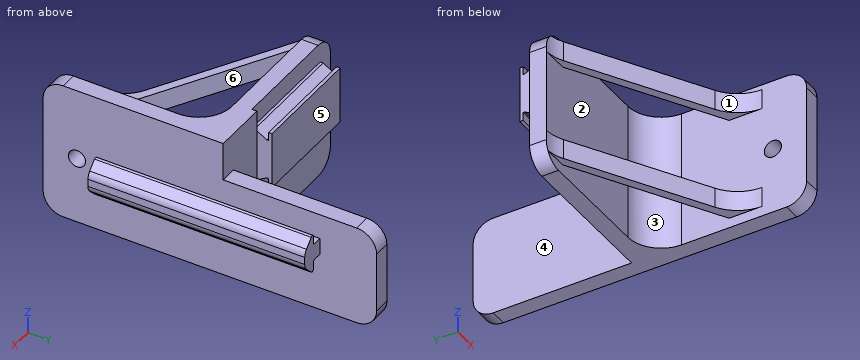
```python
from build123d import *

# Parameters (mm, degrees)
BOSS_EXTRUDE5_DEPTH  = 50
SKETCH11_W           = 41.5
SKETCH11_H           = 100
BOSS_EXTRUDE6_DEPTH  = 5
SKETCH12_W           = 41.5
SKETCH12_H           = 5
BOSS_EXTRUDE8_DEPTH  = 55
SKETCH13_W           = 11.5
SKETCH13_H           = 47.5
CUT_EXTRUDE1_DEPTH   = 55
BOSS_EXTRUDE9_DEPTH  = 6
FILLET7_R            = 12
FILLET7_OF_MIRROR1_R = 12
FILLET8_R            = 6
BOSS_EXTRUDE10_START = 8
BOSS_EXTRUDE10_DEPTH = 8
FILLET12_R           = 10
BOSS_EXTRUDE11_DEPTH = 57
SKETCH16_R           = 2.575
CUT_EXTRUDE2_DEPTH   = 10
SKETCH17_W           = 27.480150942
SKETCH17_H           = 1.5
BOSS_EXTRUDE12_DEPTH = 11.5
SKETCH18_W           = 11.5
SKETCH18_H           = 1.5
BOSS_EXTRUDE13_DEPTH = 5
BOSS_EXTRUDE14_START = -5
BOSS_EXTRUDE14_DEPTH = 33.5


with BuildPart() as part:
    # Sketch9 → Boss-Extrude5 (new body)
    with BuildSketch(Plane(origin=(0, 245, 0), x_dir=(1, 0, 0), z_dir=(0, 1, 0))):
        with BuildLine():
            Line((389.629800237, -111.599739584), (387.629800237, -111.599739584))
            Line((387.629800237, -111.599739584), (387.629800237, -106.649739584))
            Line((387.629800237, -106.649739584), (389.629800237, -106.649739584))
            Line((389.629800237, -106.649739584), (390.329799474, -106.649739584))
            ThreePointArc((390.329799474, -106.649739584), (390.605571069, -106.535511279), (390.719799474, -106.259739725))
            Line((390.719799474, -106.259739725), (390.719800256, -104.090618139))
            ThreePointArc((390.719800256, -104.090618139), (391.145748802, -103.453141463), (391.897703935, -103.602714709))
            Line((391.897703935, -103.602714709), (394.237480965, -105.942491739))
            ThreePointArc((394.237480965, -105.942491739), (394.868289671, -106.886563682), (395.089800232, -108.000172467))
            Line((395.089800232, -108.000172467), (395.089800237, -110.249306685))
            ThreePointArc((395.089800237, -110.249306685), (394.868289678, -111.362915477), (394.23748097, -112.306987424))
            Line((394.23748097, -112.306987424), (391.897703941, -114.646764454))
            ThreePointArc((391.897703941, -114.646764454), (391.145748809, -114.7963377), (390.719800262, -114.158861025))
            Line((390.719800262, -114.158861025), (390.719799474, -111.989739443))
            ThreePointArc((390.719799474, -111.989739443), (390.605571069, -111.71396789), (390.329799474, -111.599739584))
            Line((390.329799474, -111.599739584), (389.629800237, -111.599739584))
        make_face()
    extrude(amount=-BOSS_EXTRUDE5_DEPTH)

    # Sketch11 → Boss-Extrude6 (add)
    with BuildSketch(Plane.ZY.offset(-387.629800242)):
        with Locations((109.874739584, 220)):
            Rectangle(SKETCH11_W, SKETCH11_H)
    extrude(amount=BOSS_EXTRUDE6_DEPTH)

    # Sketch12 → Boss-Extrude8 (add)
    with BuildSketch(Plane.ZY.offset(-387.629800242)):
        with Locations((109.874739584, 220)):
            Rectangle(SKETCH12_W, SKETCH12_H)
    extrude(amount=BOSS_EXTRUDE8_DEPTH)

    # Sketch13 → Cut-Extrude1 (cut)
    with BuildSketch(Plane.ZY.offset(-387.629800242)):
        with Locations((124.874739584, 246.25)):
            Rectangle(SKETCH13_W, SKETCH13_H)
    extrude(amount=CUT_EXTRUDE1_DEPTH, mode=Mode.SUBTRACT)

    # Sketch15 → Boss-Extrude9 (add)
    with BuildSketch(Plane.XY.offset(129.124739584)):
        Polygon((335.629800242, 217.5), (382.629800242, 190.364537348), (382.629800242, 193.251288694), (340.629800242, 217.5), align=None)
    boss_extrude9 = extrude(amount=-BOSS_EXTRUDE9_DEPTH)

    # Fillet7
    # the kernel refuses this fillet: 12 mm, written as the material it adds along each edge
    with BuildSketch(Plane(origin=(335.629800242, 217.5, 129.124739584), x_dir=(-1, 0, 0), z_dir=(0, 0, -1))) as fillet7_piece_1:
        with BuildLine():
            CenterArc((3.218847051, -11.998004249), FILLET7_R, 91.044975628, 28.955024372)
            Line((-2.781152949, -1.605699404), (-2.901152949, -1.397853307))
            Line((-2.901152949, -1.397853307), (-0.12, 0.207846097))
            Line((-0.12, 0.207846097), (0, 0.24))
            ThreePointArc((0, 0.24), (1.5, 0.24), (2.995623059, 0.239960085))
            Line((2.995623059, 0.239960085), (3, 0))
        make_face()
    extrude(amount=6)
    with BuildSketch(Plane(origin=(382.629800242, 190.364537348, 129.124739584), x_dir=(0, -1, 0), z_dir=(0, 0, -1))) as fillet7_piece_2:
        with BuildLine():
            CenterArc((FILLET7_R * 0.57735026919, FILLET7_R), FILLET7_R, 210, 60)
            Line((-FILLET7_R * 0.288675134595, FILLET7_R * 0.5), (-FILLET7_R * 0.305995642671, FILLET7_R * 0.49))
            Line((-FILLET7_R * 0.305995642671, FILLET7_R * 0.49), (-FILLET7_R * 0.0115470053838, -FILLET7_R * 0.02))
            Line((-FILLET7_R * 0.0115470053838, -FILLET7_R * 0.02), (FILLET7_R * 0.57735026919, -FILLET7_R * 0.02))
            Line((FILLET7_R * 0.57735026919, -FILLET7_R * 0.02), (FILLET7_R * 0.57735026919, 0))
        make_face()
    extrude(amount=6)

    # Mirror1: Boss-Extrude9 across plane
    add(boss_extrude9.mirror(Plane.XY.offset(110.624739584)))

    # Fillet7 of Mirror1
    # the kernel refuses this fillet: 12 mm, written as the material it adds along each edge
    with BuildSketch(Plane(origin=(335.629800242, 217.5, 92.124739584), x_dir=(-1, 0, 0), z_dir=(0, 0, 1))) as fillet7_of_mirror1_piece_1:
        with BuildLine():
            CenterArc((3.218847051, 11.998004249), FILLET7_OF_MIRROR1_R, 240, 28.955024372)
            Line((-2.781152949, 1.605699404), (-2.901152949, 1.397853307))
            Line((-2.901152949, 1.397853307), (-0.12, -0.207846097))
            Line((-0.12, -0.207846097), (0, -0.24))
            ThreePointArc((0, -0.24), (1.5, -0.24), (2.995623059, -0.239960085))
            Line((2.995623059, -0.239960085), (3, 0))
        make_face()
    extrude(amount=6)
    with BuildSketch(Plane(origin=(382.629800242, 190.364537348, 92.124739584), x_dir=(0, -1, 0), z_dir=(0, 0, 1))) as fillet7_of_mirror1_piece_2:
        with BuildLine():
            CenterArc((FILLET7_OF_MIRROR1_R * 0.57735026919, -FILLET7_OF_MIRROR1_R), FILLET7_OF_MIRROR1_R, 90, 60)
            Line((-FILLET7_OF_MIRROR1_R * 0.288675134595, -FILLET7_OF_MIRROR1_R * 0.5), (-FILLET7_OF_MIRROR1_R * 0.305995642671, -FILLET7_OF_MIRROR1_R * 0.49))
            Line((-FILLET7_OF_MIRROR1_R * 0.305995642671, -FILLET7_OF_MIRROR1_R * 0.49), (-FILLET7_OF_MIRROR1_R * 0.0115470053838, FILLET7_OF_MIRROR1_R * 0.02))
            Line((-FILLET7_OF_MIRROR1_R * 0.0115470053838, FILLET7_OF_MIRROR1_R * 0.02), (FILLET7_OF_MIRROR1_R * 0.57735026919, FILLET7_OF_MIRROR1_R * 0.02))
            Line((FILLET7_OF_MIRROR1_R * 0.57735026919, FILLET7_OF_MIRROR1_R * 0.02), (FILLET7_OF_MIRROR1_R * 0.57735026919, 0))
        make_face()
    extrude(amount=6)

    # Fillet8
    # the kernel refuses this fillet: 6 mm, written as the material it takes off along each edge
    with BuildSketch(Plane(origin=(402.629800242, 270, 89.124739584), x_dir=(0, 0, 1), z_dir=(-1, 0, 0)), Plane(origin=(332.629800242, 237.5, 89.124739584), x_dir=(0, 0, 1), z_dir=(0, -1, 0)), Plane(origin=(402.629800242, 270, 119.124739584), x_dir=(0, -1, 0), z_dir=(-1, 0, 0))) as fillet8_piece_1:
        with BuildLine():
            CenterArc((FILLET8_R, -FILLET8_R), FILLET8_R, 90, 90)
            Line((0, -FILLET8_R), (0, 0))
            Line((0, 0), (FILLET8_R, 0))
        make_face()
    extrude(amount=35, mode=Mode.SUBTRACT)
    with BuildSketch(Plane(origin=(402.629800242, 170, 89.124739584), x_dir=(0, 0, 1), z_dir=(-1, 0, 0)), Plane(origin=(402.629800242, 170, 130.624739584), x_dir=(0, 1, 0), z_dir=(-1, 0, 0)), Plane(origin=(332.629800242, 202.5, 130.624739584), x_dir=(1, 0, 0), z_dir=(0, 1, 0))) as fillet8_piece_2:
        with BuildLine():
            CenterArc((FILLET8_R, FILLET8_R), FILLET8_R, 180, 90)
            Line((0, FILLET8_R), (0, 0))
            Line((0, 0), (FILLET8_R, 0))
        make_face()
    extrude(amount=35, mode=Mode.SUBTRACT)

    # Sketch9<2> → Boss-Extrude10 (add)
    with BuildSketch(Plane(origin=(0, 245, 0), x_dir=(1, 0, 0), z_dir=(0, 1, 0)).offset(BOSS_EXTRUDE10_START)):
        with BuildLine():
            Line((389.629800237, -111.599739584), (387.629800237, -111.599739584))
            Line((387.629800237, -111.599739584), (387.629800237, -106.649739584))
            Line((387.629800237, -106.649739584), (389.629800237, -106.649739584))
            Line((389.629800237, -106.649739584), (390.329799474, -106.649739584))
            ThreePointArc((390.329799474, -106.649739584), (390.605571069, -106.535511279), (390.719799474, -106.259739725))
            Line((390.719799474, -106.259739725), (390.719800256, -104.090618139))
            ThreePointArc((390.719800256, -104.090618139), (391.145748802, -103.453141463), (391.897703935, -103.602714709))
            Line((391.897703935, -103.602714709), (394.237480965, -105.942491739))
            ThreePointArc((394.237480965, -105.942491739), (394.868289671, -106.886563682), (395.089800232, -108.000172467))
            Line((395.089800232, -108.000172467), (395.089800237, -110.249306685))
            ThreePointArc((395.089800237, -110.249306685), (394.868289678, -111.362915477), (394.23748097, -112.306987424))
            Line((394.23748097, -112.306987424), (391.897703941, -114.646764454))
            ThreePointArc((391.897703941, -114.646764454), (391.145748809, -114.7963377), (390.719800262, -114.158861025))
            Line((390.719800262, -114.158861025), (390.719799474, -111.989739443))
            ThreePointArc((390.719799474, -111.989739443), (390.605571069, -111.71396789), (390.329799474, -111.599739584))
            Line((390.329799474, -111.599739584), (389.629800237, -111.599739584))
        make_face()
    extrude(amount=-BOSS_EXTRUDE10_DEPTH)

    # Fillet12
    fillet12_edges = [part.edges().sort_by_distance(p)[0] for p in [
        (382.629800242, 217.5, 109.874739584),
    ]]
    fillet(fillet12_edges, radius=FILLET12_R)

    # Sketch9<3> → Boss-Extrude11 (add)
    with BuildSketch(Plane(origin=(0, 245, 0), x_dir=(1, 0, 0), z_dir=(0, 1, 0))):
        with BuildLine():
            Line((389.629800237, -111.599739584), (387.629800237, -111.599739584))
            Line((387.629800237, -111.599739584), (387.629800237, -106.649739584))
            Line((387.629800237, -106.649739584), (389.629800237, -106.649739584))
            Line((389.629800237, -106.649739584), (390.329799474, -106.649739584))
            ThreePointArc((390.329799474, -106.649739584), (390.605571069, -106.535511279), (390.719799474, -106.259739725))
            Line((390.719799474, -106.259739725), (390.719800256, -104.090618139))
            ThreePointArc((390.719800256, -104.090618139), (391.145748802, -103.453141463), (391.897703935, -103.602714709))
            Line((391.897703935, -103.602714709), (394.237480965, -105.942491739))
            ThreePointArc((394.237480965, -105.942491739), (394.868289671, -106.886563682), (395.089800232, -108.000172467))
            Line((395.089800232, -108.000172467), (395.089800237, -110.249306685))
            ThreePointArc((395.089800237, -110.249306685), (394.868289678, -111.362915477), (394.23748097, -112.306987424))
            Line((394.23748097, -112.306987424), (391.897703941, -114.646764454))
            ThreePointArc((391.897703941, -114.646764454), (391.145748809, -114.7963377), (390.719800262, -114.158861025))
            Line((390.719800262, -114.158861025), (390.719799474, -111.989739443))
            ThreePointArc((390.719799474, -111.989739443), (390.605571069, -111.71396789), (390.329799474, -111.599739584))
            Line((390.329799474, -111.599739584), (389.629800237, -111.599739584))
        make_face()
    extrude(amount=-BOSS_EXTRUDE11_DEPTH)

    # Sketch16 → Cut-Extrude2 (cut)
    with BuildSketch(Plane.ZY.offset(-382.629800242)):
        with Locations((109.124739584, 180.133064736)):
            Circle(SKETCH16_R)
    extrude(amount=-CUT_EXTRUDE2_DEPTH, mode=Mode.SUBTRACT)

    # Sketch17 → Boss-Extrude12 (add)
    with BuildSketch(Plane(origin=(371.129800242, 0, 0), x_dir=(0, 0, -1), z_dir=(1, 0, 0))):
        with Locations((-116.884664113, 223.25)):
            Rectangle(SKETCH17_W, SKETCH17_H)
    extrude(amount=BOSS_EXTRUDE12_DEPTH)

    # Sketch18 → Boss-Extrude13 (add)
    with BuildSketch(Plane(origin=(382.629800242, 0, 0), x_dir=(0, 0, -1), z_dir=(1, 0, 0))):
        with Locations((-124.874739584, 223.25)):
            Rectangle(SKETCH18_W, SKETCH18_H)
    extrude(amount=BOSS_EXTRUDE13_DEPTH)

    # Sketch19 → Boss-Extrude14 (add)
    with BuildSketch(Plane.ZY.offset(-332.629800242).offset(BOSS_EXTRUDE14_START)):
        Polygon((125.144664113, 227.49), (125.144664113, 228.51), (108.124664113, 228.51), (108.124664113, 227.49), (110.624664113, 227.49), (110.624664113, 227.002681543), (108.524291386, 223.367942117), (108.524291386, 222.5), (124.745036841, 222.5), (124.745036841, 223.367942117), (122.644664113, 227.002681543), (122.644664113, 227.49), align=None)
    extrude(amount=-BOSS_EXTRUDE14_DEPTH)


solid = part.part
```
Geometry: final body of the model. Coordinates: model frame, mm. Face numbers are marked on the shaded views. A direction names the side the tool comes from. Coordinates: 2 decimals unless noted, no trailing zeros. Loops run counter-clockwise (first coordinate to the right, second up) from the corner with the lowest first, then second, coordinate; pieces in that order, holes last. Notation, with made-up numbers: (8, 89.25) -> (15, 89.25) arc R26 ccw to (15, 105.25) -> close; hole circle Ø11 at (75.25, 11.5). An arc over 180 degrees is marked (long way). Use a Markdown table: item, result. Add a question column.
(1) Mould query, pull axis Y, two halves, no side actions, for the marked faces 4, 5 and 6. Classes: pulls with the +Y half, pulls with the -Y half, needs draft (parallel to the pull), parting line crosses it, or undercut.
(2) Section query B-B, the plane y = 206. Return loops of the section in (x, z), plus the area to 3 significant figures.
(3) Pin query (flat end, axial travel): pin 1 Ø1.3 at (x, y) = (389.5, 209) entering from +Z; pin 2 Ø1 at (x, y) = (388.5, 218) entering from -Z; pin 3 Ø6 at (x, z) = (390.5, 109.5) entering from -Y; pin 4 Ø0.8 at (x, y) = (359, 228) entering from +Z. Return the tip coordinate at first contact, or that it passes through.
(4) Line query: line 1 along X through (y, z) = (240.5, 109); line 2 along Y through (x, z) = (367, 100); line 3 along X through (y, z) = (257, 99). Output: solid intervals per line, ascending.
(5) Section query C-C, the plane y = 231.5. Return loops of the section in (x, z).
(6) Section query A-A, the plane x = 363.5. Return loops of the section in (y, z).
(7) Access query for the marked faces 1, 2 and 3. Directions: +Z, -Z, +X, -X, +Y, -Y. A direction counts if a zero-diameter tool reaches every point of the face in a straight line with its end or side. Return the directions, or none.
(8) Section query D-D, the plane z = 99.5. Return loops of the section in (x, y).
Answer:
| question | item | result |
|---|---|---|
| 1 | face 4 | needs draft |
| 1 | face 5 | pulls with the +Y half |
| 1 | face 6 | undercut |
| 2 | outline | (355.55, 92.12) -> (360.55, 92.12) -> (360.55, 98.12) -> (355.55, 98.12) -> close; (355.55, 123.12) -> (360.55, 123.12) -> (360.55, 129.12) -> (355.55, 129.12) -> close; (382.63, 89.12) -> (387.63, 89.12) -> (387.63, 106.65) -> (390.33, 106.65) arc R0.39 cw to (390.72, 106.26) -> (390.72, 104.09) arc R0.69 ccw to (391.9, 103.6) -> (394.24, 105.94) arc R2.91 ccw to (395.09, 108) -> (395.09, 110.25) arc R2.91 ccw to (394.24, 112.31) -> (391.9, 114.65) arc R0.69 ccw to (390.72, 114.16) -> (390.72, 111.99) arc R0.39 cw to (390.33, 111.6) -> (387.63, 111.6) -> (387.63, 130.62) -> (382.63, 130.62) -> close |
| 2 | area | 321 mm^2 |
| 3 | pin 1 | stops at z = 111.6 |
| 3 | pin 2 | stops at z = 106.65 |
| 3 | pin 3 | stops at y = 170 |
| 3 | pin 4 | stops at z = 125.14 |
| 4 | line 1 | x = 382.63 to 395.09 |
| 4 | line 2 | y = 217.5 to 222.5 |
| 4 | line 3 | x = 382.63 to 387.63 |
| 5 | outline | (382.63, 89.12) -> (387.63, 89.12) -> (387.63, 106.65) -> (390.33, 106.65) arc R0.39 cw to (390.72, 106.26) -> (390.72, 104.09) arc R0.69 ccw to (391.9, 103.6) -> (394.24, 105.94) arc R2.91 ccw to (395.09, 108) -> (395.09, 110.25) arc R2.91 ccw to (394.24, 112.31) -> (391.9, 114.65) arc R0.69 ccw to (390.72, 114.16) -> (390.72, 111.99) arc R0.39 cw to (390.33, 111.6) -> (387.63, 111.6) -> (387.63, 119.12) -> (382.63, 119.12) -> close |
| 6 | outline | (201.41, 92.12) -> (204.3, 92.12) -> (204.3, 98.12) -> (201.41, 98.12) -> close; (201.41, 123.12) -> (204.3, 123.12) -> (204.3, 129.12) -> (201.41, 129.12) -> close; (217.5, 89.12) -> (222.5, 89.12) -> (222.5, 108.52) -> (223.37, 108.52) -> (227, 110.62) -> (227.49, 110.62) -> (227.49, 108.12) -> (228.51, 108.12) -> (228.51, 125.14) -> (227.49, 125.14) -> (227.49, 122.64) -> (227, 122.64) -> (223.37, 124.75) -> (222.5, 124.75) -> (222.5, 130.62) -> (217.5, 130.62) -> close |
| 7 | face 1 | +Z, -Z, -X, -Y |
| 7 | face 2 | none |
| 7 | face 3 | +Z, -Z |
| 8 | outline | (332.63, 217.5) -> (372.63, 217.5) arc R10 cw to (382.63, 207.5) -> (382.63, 170) -> (387.63, 170) -> (387.63, 270) -> (382.63, 270) -> (382.63, 222.5) -> (332.63, 222.5) -> close |
